Part model, mm, in its own coordinate system. Face numbers are marked on the shaded views. A direction names the side the tool comes from. Round coordinates to 2 decimals unless told otherwise and drop trailing zeros. Loops run counter-clockwise (first coordinate to the right, second up) from the corner with the lowest first, then second, coordinate; pieces in that order, holes last.
(1) Cut at A-A on x = 4.5. List the corners of the cut face in (y, z) (3 decimals), then the cut area to 3 significant figures.
(2) Mould opens along X. For the marked faces 3, 4, 5 and 6 say: +X half, -X half, draft (parallel to the pull), parting line (faces both ways), or undercut.
(3) Tool access for the marked faces 1 and 2: list every direction of +Z, -Z, +X, -X, +Y, -Y with a clear straight run to the whole face (end or side of a thin tool).
(4) Flat gauge pin, fed straight in: pin 1 (3.5 mm diameter, centred on x = 0, y = 0, fed in from +Z). Where does the tip first touch, or does it go through?
(5) Probe probe 1 along Y at (x, z) = (0, 5.5); probe 2 along X at (y, z) = (-8.7, 0). List the from-to ranges inside material, lowest first.
from build123d import *

# Parameters (mm, degrees)
F0_W     = 17.78
F0_H     = 17.78
F1_DEPTH = 8.89
F5_D     = 0.508
F5_DEPTH = 0.508
F5_TIP   = 0.1526185972
F6_D     = 4.0386
F6_DEPTH = 10.16
F6_TIP   = 1.213317848
F7_D     = 6.35
F7_DEPTH = 10.16
F7_TIP   = 1.9077324654


with BuildPart() as f1:
    # F0 (on Front) → F1 (new body, symmetric)
    with BuildSketch(Plane.XZ):
        Rectangle(F0_W, F0_H)
    extrude(amount=F1_DEPTH, both=True)

    # F5
    with Locations(Plane.XZ.offset(8.89)):
        with Locations((0, 0)):
            Hole(F5_D / 2, depth=F5_DEPTH)
            with Locations((0, 0, -(F5_DEPTH + F5_TIP / 2))):  # 118° drill point
                Cone(0, F5_D / 2, F5_TIP, mode=Mode.SUBTRACT)

    # F6
    with Locations(Plane.XY.offset(8.89)):
        with Locations((0, 0)):
            Hole(F6_D / 2, depth=F6_DEPTH)
            with Locations((0, 0, -(F6_DEPTH + F6_TIP / 2))):  # 118° drill point
                Cone(0, F6_D / 2, F6_TIP, mode=Mode.SUBTRACT)

    # F7
    with Locations(Plane.YZ.offset(8.89)):
        with Locations((0, 0)):
            Hole(F7_D / 2, depth=F7_DEPTH)
            with Locations((0, 0, -(F7_DEPTH + F7_TIP / 2))):  # 118° drill point
                Cone(0, F7_D / 2, F7_TIP, mode=Mode.SUBTRACT)


solid = f1.part
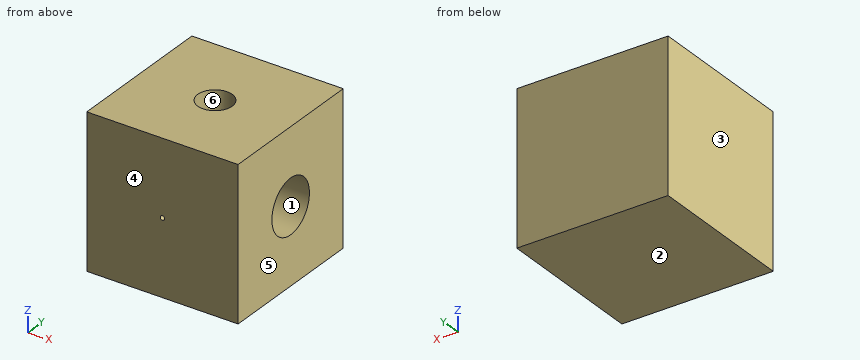
Final values:
1. outline: (-8.89, -8.89) - (8.89, -8.89) - (8.89, 8.89) - (-8.89, 8.89) - close; hole circle Ø6.35 at (0, 0)
1. area: 284 mm2
2. face 3: -X half
2. face 4: draft
2. face 5: +X half
2. face 6: undercut
3. face 1: +X
3. face 2: -Z, +X, -X, +Y, -Y
4. pin 1: stops at z = -2.38
5. probe 1: y = -8.89 to -2.02, 2.02 to 8.89
5. probe 2: x = -8.89 to -0.25, 0.25 to 8.89
